Source: CAD feature listing. Evaluate the final solid. Frame: model axes, mm. Round coordinates to 2 decimals unless told otherwise and drop trailing zeros. Order: outer loops, then holes, each group sorted by start corner. A loop starts at its lowest first (then second) coordinate and runs counter-clockwise, first axis right, second up. Notation, with made-up numbers: (59.25, 50.5) -> (117.25, 50.5) arc R8 cw to (117.25, 63.5) -> close; hole circle Ø1 at (59, -1.5). An arc over 180 degrees is marked (long way). One line per item, written item: value. Start each with the question number.
1) Section C-C (z = 0.9). State how many separate pieces and enclosed holes the cut face has, and give its area (3 significant figures).
2) Pin query (flat end, axial travel): P1, Ø0.9, axis at y = 148.5, z = 1, coming from the -X side; P2, Ø1, axis at x = 74.5, y = -52, coming from the -Z side. Return the tip coordinate at first contact, or that it passes through.
3) Section A-A (y = 101.5). Return the cut outline in (x, z) (3 decimals).
4) Section B-B (x = 144). Return the cut outline in (y, z) (3 decimals), and give its area (4 significant figures).
5) Ray query, L1, parallel to Y at x = 52, z = 0.7 (3 decimals); L2, parallel to X at y = -39.5, z = 0.55 (3 decimals); L3, parallel to X at y = -143.5, z = 2. Return the intervals inside material, ascending.
```python
from build123d import *

# Parameters (mm, degrees)
F1_DEPTH = 3
F2_W     = 40
F2_H     = 3.25
F2_W_2   = 3.25
F2_H_2   = 30
F3_DEPTH = 3


with BuildPart() as f1:
    # F0 (on Top) → F1 (new body)
    with BuildSketch(Plane.XY):
        with BuildLine():
            Line((190, 160), (-190, 160))
            ThreePointArc((-190, 160), (-204.142136, 154.142136), (-210, 140))
            Line((-210, 140), (-210, -140))
            ThreePointArc((-210, -140), (-204.142136, -154.142136), (-190, -160))
            Line((-190, -160), (190, -160))
            ThreePointArc((190, -160), (204.142136, -154.142136), (210, -140))
            Line((210, -140), (210, 140))
            ThreePointArc((210, 140), (204.142136, 154.142136), (190, 160))
        make_face()
    extrude(amount=F1_DEPTH)

    # F2 (on face) → F3 (cut)
    with BuildSketch(Plane.XY.offset(3)):
        with Locations((-140, 148.5)):
            Rectangle(F2_W, F2_H)
        with Locations((-60, 148.5)):
            Rectangle(F2_W, F2_H)
        with Locations((60, 148.5)):
            Rectangle(F2_W, F2_H)
        with Locations((140, 148.5)):
            Rectangle(F2_W, F2_H)
        with Locations((198.5, 105)):
            Rectangle(F2_W_2, F2_H_2)
        with Locations((198.5, 45)):
            Rectangle(F2_W_2, F2_H_2)
        with Locations((198.5, -45)):
            Rectangle(F2_W_2, F2_H_2)
        with Locations((-198.5, 105)):
            Rectangle(F2_W_2, F2_H_2)
        with Locations((-198.5, 45)):
            Rectangle(F2_W_2, F2_H_2)
        with Locations((-198.5, -45)):
            Rectangle(F2_W_2, F2_H_2)
        with Locations((-198.5, -105)):
            Rectangle(F2_W_2, F2_H_2)
        with Locations((-140, -148.5)):
            Rectangle(F2_W, F2_H)
        with Locations((-60, -148.5)):
            Rectangle(F2_W, F2_H)
        with Locations((60, -148.5)):
            Rectangle(F2_W, F2_H)
        with Locations((140, -148.5)):
            Rectangle(F2_W, F2_H)
        with Locations((198.5, -105)):
            Rectangle(F2_W_2, F2_H_2)
    extrude(amount=-F3_DEPTH, mode=Mode.SUBTRACT)


solid = f1.part
```
Findings:
1. separate pieces: 1
1. enclosed holes: 16
1. area: 132,000 mm2
2. P1: x = -208.31
2. P2: z = 0
3. outline: (-210, 0) -> (-200.125, 0) -> (-200.125, 3) -> (-210, 3) -> close; (-196.875, 0) -> (196.875, 0) -> (196.875, 3) -> (-196.875, 3) -> close; (200.125, 0) -> (210, 0) -> (210, 3) -> (200.125, 3) -> close
4. outline: (-160, 0) -> (-150.125, 0) -> (-150.125, 3) -> (-160, 3) -> close; (-146.875, 0) -> (146.875, 0) -> (146.875, 3) -> (-146.875, 3) -> close; (150.125, 0) -> (160, 0) -> (160, 3) -> (150.125, 3) -> close
4. area: 940.5 mm2
5. L1: -160 to -150.125, -146.875 to 146.875, 150.125 to 160
5. L2: -210 to -200.125, -196.875 to 196.875, 200.125 to 210
5. L3: -209.69 to 209.69
